from build123d import *

# Parameters (mm, degrees)
BOSS_EXTRU_2_DEPTH      = 10
ENL_V_MAT_EXTRU_1_REACH = 20.547
ESQUISSE3_R             = 2
ENL_V_MAT_EXTRU_2_REACH = 20.547
ESQUISSE4_R             = 2
CONG_1_R                = 2
CONG_2_R                = 0.5


with BuildPart() as part:
    # Esquisse2 → Boss.-Extru.2 (new body)
    with BuildSketch(Plane.XY):
        Polygon((0, 12), (12, 12), (12, 0), (10, 0), (10, 10), (0, 10), align=None)
    extrude(amount=BOSS_EXTRU_2_DEPTH)

    # Esquisse3 → Enlèv. mat.-Extru.1 (cut, up to next)
    with BuildSketch(Plane.ZY.offset(-10), mode=Mode.PRIVATE) as enl_v_mat_extru_1_sk1:
        with Locations(Location((5, 4.5, 0), (0, 0, 270))):
            Circle(ESQUISSE3_R)
    enl_v_mat_extru_1_tool1 = extrude(enl_v_mat_extru_1_sk1.sketch, amount=-ENL_V_MAT_EXTRU_1_REACH, mode=Mode.PRIVATE) & part.part
    add(enl_v_mat_extru_1_tool1.solids().sort_by_distance((10, 4.5, 5))[0], mode=Mode.SUBTRACT)

    # Esquisse4 → Enlèv. mat.-Extru.2 (cut, up to next)
    with BuildSketch(Plane.XZ.offset(-10), mode=Mode.PRIVATE) as enl_v_mat_extru_2_sk1:
        with Locations((4.5, 5)):
            Circle(ESQUISSE4_R)
    enl_v_mat_extru_2_tool1 = extrude(enl_v_mat_extru_2_sk1.sketch, amount=-ENL_V_MAT_EXTRU_2_REACH, mode=Mode.PRIVATE) & part.part
    add(enl_v_mat_extru_2_tool1.solids().sort_by_distance((4.5, 10, 5))[0], mode=Mode.SUBTRACT)

    # Congé1
    cong_1_edges = [part.edges().sort_by_distance(p)[0] for p in [
        (12, 12, 5),
    ]]
    fillet(cong_1_edges, radius=CONG_1_R)

    # Congé2
    cong_2_edges = [part.edges().sort_by_distance(p)[0] for p in [
        (10, 10, 5),
    ]]
    fillet(cong_2_edges, radius=CONG_2_R)


solid = part.part
Geometry: final body of the model. Coordinates: model frame, mm. A direction names the side the tool comes from. Give positions to 0.01 mm unless a question says otherwise; leave off trailing zeros. Order: outer loops, then holes, each group sorted by start corner. A loop starts at its lowest first (then second) coordinate and runs counter-clockwise, first axis right, second up. Notation, with made-up numbers: (-40, -11.5) -> (-15, -11.5) arc R18 cw to (-15, 21.5) -> close; hole circle Ø2 at (60.25, -17.75). An arc over 180 degrees is marked (long way). Answer as a JSON object with one key per item and string values.
Q1. First-contact query: pin 1 (1 mm diameter, centred on x = 3, z = 2, fed in from -Y); pin 2 (5 mm diameter, centred on y = 4.5, z = 8, fed in from -X); pin 3 (3 mm diameter, centred on y = 4.5, z = 5, fed in from -X). Flat tips, straight axial feed; report the tip coordinate or a pass-through.
Entries:
{"pin 1": "stops at y = 10", "pin 2": "stops at x = 10", "pin 3": "passes through"}
Q2. Section D-D (z = 8). Output: boundary loops of the cut face in (x, y), plus the area to 3 significant figures.
Entries:
{"outline": "(0, 10) -> (9.5, 10) arc R0.5 cw to (10, 9.5) -> (10, 0) -> (12, 0) -> (12, 10) arc R2 ccw to (10, 12) -> (0, 12) -> close", "area": "43.2 mm^2"}
Q3. Material intervals for probe 1 along Z at (x, y) = (10.5, 4.5); probe 2 along Y at (x, z) = (8, 4), sorted ascending.
Entries:
{"probe 1": "z = 0 to 3, 7 to 10", "probe 2": "y = 10 to 12"}
Q4. Section A-A (x = 4.5). Output: boundary loops of the cut face in (y, z).
Entries:
{"outline": "(10, 0) -> (12, 0) -> (12, 3) -> (10, 3) -> close; (10, 7) -> (12, 7) -> (12, 10) -> (10, 10) -> close"}
Q5. Draft query along Z for faces 3 (the cylindrical face through (2.502, 10.986, 5.088)), 4 (the flat face through (12, 7, 5)). Return one class per face: released by +Z, released by -Z, zero draft, split by the parting line, or undercut.
Entries:
{"face 3": "undercut", "face 4": "zero draft"}
Q6. Access query for faces 1 (the flat face through (10, 7, 5)), 2 (the flat face through (0, 11, 5)). Directions: +Z, -Z, +X, -X, +Y, -Y. A direction counts if a zero-diameter tool reaches every point of the face in a straight line with its end or side. Return the directions, or none.
Entries:
{"face 1": "+Z, -Z, -X, -Y", "face 2": "+Z, -Z, -X, +Y, -Y"}
Q7. Section B-B (z = 5). Output: boundary loops of the cut face in (x, y).
Entries:
{"outline": "(0, 10) -> (2.5, 10) -> (2.5, 12) -> (0, 12) -> close; (6.5, 10) -> (9.5, 10) arc R0.5 cw to (10, 9.5) -> (10, 6.5) -> (12, 6.5) -> (12, 10) arc R2 ccw to (10, 12) -> (6.5, 12) -> close; (10, 0) -> (12, 0) -> (12, 2.5) -> (10, 2.5) -> close"}
